```python
from build123d import *

# Parameters (mm, degrees)
SKETCH1_R                = 1.75
BOSS_EXTRUDE1_DEPTH      = 3
SKETCH2_R                = 1.4
BOSS_EXTRUDE2_DEPTH      = 3
BOSS_EXTRUDE2_DEPTH_BACK = 3
FILLET1_R                = 1


with BuildPart() as part:
    # Sketch1 → Boss-Extrude1 (new body)
    with BuildSketch(Plane.XY):
        with BuildLine():
            Line((-12, 5), (12, 5))
            ThreePointArc((12, 5), (17, 0), (12, -5))
            Line((12, -5), (-12, -5))
            ThreePointArc((-12, -5), (-17, 0), (-12, 5))
        make_face()
        with Locations((-7, 0)):
            Circle(SKETCH1_R, mode=Mode.SUBTRACT)
        with Locations((-12, 0)):
            Circle(SKETCH1_R, mode=Mode.SUBTRACT)
        with Locations((12, 0)):
            Circle(SKETCH1_R, mode=Mode.SUBTRACT)
        with Locations((7, 0)):
            Circle(SKETCH1_R, mode=Mode.SUBTRACT)
    extrude(amount=BOSS_EXTRUDE1_DEPTH)

    # Sketch2 → Boss-Extrude2 (add, two sides)
    with BuildSketch(Plane.XY.offset(3)) as boss_extrude2_sk:
        with BuildLine():
            ThreePointArc((-7.961, 2.947283325), (-17, 0), (-7.961, -2.947283325))
            ThreePointArc((-7.961, -2.947283325), (-10.1, 0), (-7.961, 2.947283325))
        make_face()
        with Locations((-12, 0)):
            Circle(SKETCH2_R, mode=Mode.SUBTRACT)
        with BuildLine():
            ThreePointArc((7.961, 2.947283325), (10.1, 0), (7.961, -2.947283325))
            ThreePointArc((7.961, -2.947283325), (17, 0), (7.961, 2.947283325))
        make_face()
        with Locations((12, 0)):
            Circle(SKETCH2_R, mode=Mode.SUBTRACT)
    extrude(amount=BOSS_EXTRUDE2_DEPTH)
    extrude(boss_extrude2_sk.sketch, amount=-BOSS_EXTRUDE2_DEPTH_BACK)

    # Fillet1
    fillet1_edges = [part.edges().sort_by_distance(p)[0] for p in [
        (-7.961, -2.947283325, 4.5),
        (-7.961, 2.947283325, 4.5),
        (7.961, 2.947283325, 4.5),
        (7.961, -2.947283325, 4.5),
    ]]
    fillet(fillet1_edges, radius=FILLET1_R)


solid = part.part
```
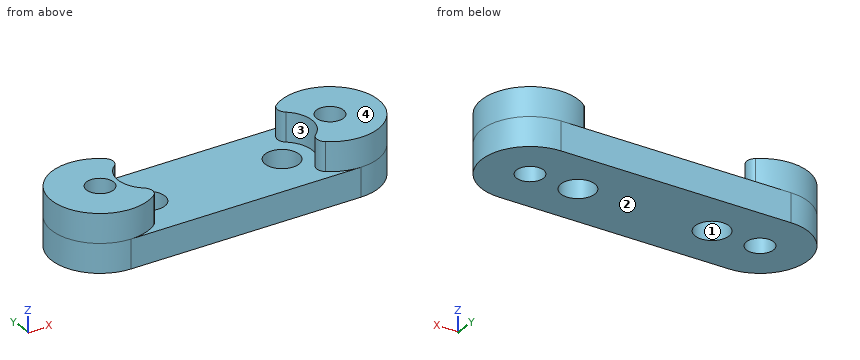
Here's how the part is built. I have some questions about the finished solid (model axes, mm). Face numbers are marked on the shaded views. A direction names the side the tool comes from. Coordinates: 2 decimals unless noted, no trailing zeros. Write each loop counter-clockwise with the first axis right and the second up, starting at its lowest first coordinate (ties: lowest second). Pieces come first, ordered by that corner, then holes. Notation, with made-up numbers: M 17,25.5 L 74,25.5 A18 cw 74,36.5 Z; hole C 29,2 d11. An arc over 180 degrees is marked long. Answer as CSV lines item,"result". Start each with the question number.
Q1. If we mould it in two halves opening along X, with no side actions, what happens to the marked faces 1 and 2? For each: pulls with the +X half, pulls with the -X half, needs draft (parallel to the pull), parting line crosses it, or undercut.
Q2. Suppose I cut it at A-A, the plane z = 1. List the corners of the cut face in (x, y) for me.
Q3. Will these pins go through, and if not, where does the flat tip stop? pin 1 Ø4 at (x, y) = (-7, 0) entering from -Z; pin 2 Ø3 at (x, y) = (7, 0) entering from -Z; pin 3 Ø4 at (x, y) = (6.5, 0) entering from +Z.
Q4. Suppose I cut it at D-D, the plane z = 3.5. State how many separate pieces and enclosed holes the cut face has, then the cut area to 3 significant figures.
Q5. For the marked faces 3 and 4, which set-ups out of +Z, -Z, +X, -X, +Y, -Y let a thin tool reach every point of the face, with its end or its side?
Q6. I need wall thicknesses on probe 1 along Y at (x, z) = (-7, 0.9); probe 2 along X at (y, z) = (0.5, 4.5); probe 3 along Y at (x, z) = (12, 1.85). Which ranges of each line are inside material? Lowest first, please. Write a range as [from, to].
Q7. Suppose I cut it at C-C, the plane y = -0.75. List the corners of the cut face in (x, z) for me.
Q8. Suppose I cut it at B-B, the plane x = 7. List the corners of the cut face in (y, z) for me, then the cut area to 3 significant figures.
Entries:
1,face 1,"undercut"
1,face 2,"needs draft"
2,outline,"M -12,-5 L 12,-5 A5 ccw 12,5 L -12,5 A5 ccw Z; hole C -12,0 d2.8; hole C -7,0 d3.5; hole C 7,0 d3.5; hole C 12,0 d2.8"
3,pin 1,"stops at z = 0"
3,pin 2,"passes through"
3,pin 3,"stops at z = 3"
4,separate pieces,"2"
4,enclosed holes,"2"
4,area,"117 mm²"
5,face 3,"+Z"
5,face 4,"+Z, +X, -X, +Y, -Y"
6,probe 1,"y = [-5, -1.75], [1.75, 5]"
6,probe 2,"x = [-16.97, -13.31], [-10.69, -10.06], [10.06, 10.69], [13.31, 16.97]"
6,probe 3,"y = [-5, -1.4], [1.4, 5]"
7,outline,"M -16.94,0 L -13.18,0 L -13.18,6 L -16.94,6 Z; M -10.82,0 L -8.58,0 L -8.58,3 L -10.01,3 L -10.01,6 L -10.82,6 Z; M -5.42,0 L 5.42,0 L 5.42,3 L -5.42,3 Z; M 8.58,0 L 10.82,0 L 10.82,6 L 10.01,6 L 10.01,3 L 8.58,3 Z; M 13.18,0 L 16.94,0 L 16.94,6 L 13.18,6 Z"
8,outline,"M -5,0 L -1.75,0 L -1.75,3 L -5,3 Z; M 1.75,0 L 5,0 L 5,3 L 1.75,3 Z"
8,area,"19.5 mm²"
